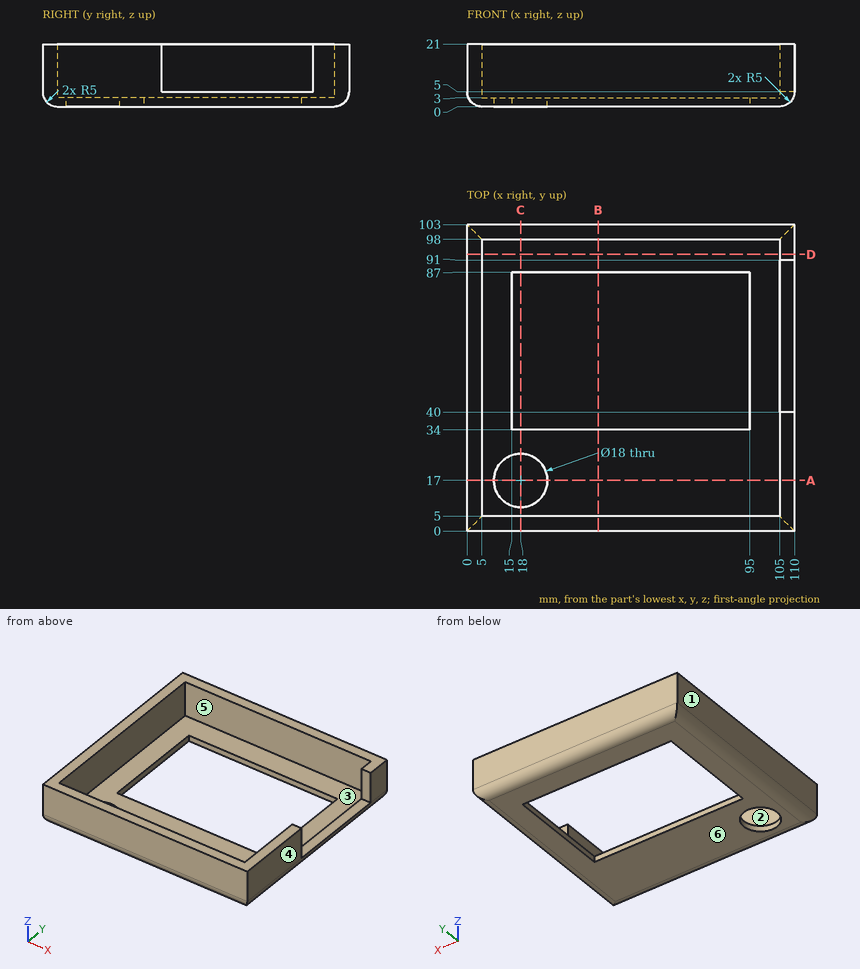
Input: dimensioned drawing with shaded views. Units: mm. Origin: part minimum x, y, z. A direction names the side the tool comes from. Round coordinates to 2 decimals unless told otherwise and drop trailing zeros. Order: outer loops, then holes, each group sorted by start corner. A loop starts at its lowest first (then second) coordinate and runs counter-clockwise, first axis right, second up. Notation, with made-up numbers: (36, -38) - (41, -38) arc R28 cw to (41, -7) - close; hole circle Ø3 at (-31, 37). An arc over 180 degrees is marked (long way). Use CSV: the item, a comma, the result in double quotes. Start each with the question number.
Q1. Section query D-D (y = 93). Return loops of the section in (x, z), and give its area (3 significant figures).
Q2. Material intervals for line 1 along Y through (x, z) = (18, 1.9); line 2 along X through (y, z) = (31, 14); line 3 along Y through (x, z) = (79.5, 19), sorted ascending. Write a range as from..to.
Q3. First-contact query: pin 1 (3.5 mm diameter, centred on y = 67, z = 1.5, fed in from -X); pin 2 (3.5 mm diameter, centred on y = 66, z = 2, fed in from +X); pin 3 (2.5 mm diameter, centred on x = 107.5, y = 73, fed in from +Z). Flat tips, straight axial feed; report the tip coordinate or a pass-through.
Q4. Section query C-C (x = 18). Return loops of the section in (y, z).
Q5. Access query for the marked faces 5 and 6. Directions: +Z, -Z, +X, -X, +Y, -Y. A direction counts if a zero-diameter tool reaches every point of the face in a straight line with its end or side. Return the directions, or none.
Q6. Section query B-B (x = 44). Return loops of the section in (y, z).
Q7. Mould query, pull axis X, two halves, no side actions, for the marked faces 1, 2, 3 and 4. Classes: +X half, -X half, draft (parallel to the pull), parting line (faces both ways), or undercut.
Q8. Section query A-A (y = 17). Return loops of the section in (x, z), and give its area (3 significant figures).
Result set:
1,outline,"(0, 5) arc R5 ccw to (5, 0) - (105, 0) arc R5 ccw to (110, 5) - (110, 21) - (105, 21) - (105, 3) - (5, 3) - (5, 21) - (0, 21) - close"
1,area,"499 mm2"
2,line 1,"y = 1.08..8, 26..34, 87..101.92"
2,line 2,"x = 0..5, 105..110"
2,line 3,"y = 0..5, 98..103"
3,pin 1,"stops at x = 0.32"
3,pin 2,"stops at x = 109.84"
3,pin 3,"stops at z = 5"
4,outline,"(0, 5) arc R5 ccw to (5, 0) - (8, 0) - (8, 3) - (5, 3) - (5, 21) - (0, 21) - close; (26, 0) - (34, 0) - (34, 3) - (26, 3) - close; (87, 0) - (98, 0) arc R5 ccw to (103, 5) - (103, 21) - (98, 21) - (98, 3) - (87, 3) - close"
5,face 5,"+Z"
5,face 6,"-Z, +X, -X, +Y, -Y"
6,outline,"(0, 5) arc R5 ccw to (5, 0) - (34, 0) - (34, 3) - (5, 3) - (5, 21) - (0, 21) - close; (87, 0) - (98, 0) arc R5 ccw to (103, 5) - (103, 21) - (98, 21) - (98, 3) - (87, 3) - close"
7,face 1,"-X half"
7,face 2,"undercut"
7,face 3,"undercut"
7,face 4,"+X half"
8,outline,"(0, 5) arc R5 ccw to (5, 0) - (9, 0) - (9, 3) - (5, 3) - (5, 21) - (0, 21) - close; (27, 0) - (105, 0) arc R5 ccw to (110, 5) - (110, 21) - (105, 21) - (105, 3) - (27, 3) - close"
8,area,"445 mm2"
